Design review of the part built by this model. Coordinates are the model's own, in mm. A direction names the side the tool comes from. Give positions to 0.01 mm unless a question says otherwise; leave off trailing zeros. Order: outer loops, then holes, each group sorted by start corner. A loop starts at its lowest first (then second) coordinate and runs counter-clockwise, first axis right, second up. Notation, with made-up numbers: (34.5, 29.5) -> (67.5, 29.5) arc R21 ccw to (67.5, 40.5) -> close; hole circle Ø10 at (-9, 83.5). An arc over 180 degrees is marked (long way). One line per item, written item: value.
Autodesk Fusion 360 part; units mm, degrees
sketch "スケッチ1" plane through (0, 0, 0) normal (0, 0, 1) x (1, 0, 0)
  line L0 (0, 45) -> (0, 0)
  line L1 (4, 10.5) -> (4, 45)
  line L2 (45, 4) -> (10.5, 4)
  line L3 (0, 0) -> (45, 0)
  arc A0 (4, 10.5) -> (10.5, 4) centre (10.5, 10.5) ccw
  line L4 (45, 0) -> (45, 4)
  line L5 (4, 45) -> (0, 45)
extrude "押し出し1" add sketch "スケッチ1" along normal blind 100
Item 1: Add section B-B on x = 16.5. Give the boundary of the cut face in (y, z).
Returned:
outline: (0, 0) -> (4, 0) -> (4, 100) -> (0, 100) -> close
Item 2: To check wall thickness, follow line 1 along X through (y, z) = (26, 80); line 2 along X through (y, z) = (9, 60). State the ranges of each line that lie inside material, in increasing order. Write a range as from..to.
Returned:
line 1: 0..4
line 2: 0..4.18
Item 3: Clearance check with flat-ended pins moving along their axes: P1, Ø4, axis at x = 26, z = 62.5, coming from the +Y side; P2, Ø10.5, axis at y = 36, z = 53, coming from the +X side; P3, Ø6, axis at y = 33.5, z = 38, coming from the -X side; P4, Ø4, axis at y = 10.5, z = 58.5, coming from the +X side. State where each tip first meets the part, or that it passes through.
Returned:
P1: y = 4
P2: x = 4
P3: x = 0
P4: x = 4.32
Item 4: Machinability: for faces 1 (the flat face through (22, 0, 49)), 2 (the flat face through (28, 4, 49)), which of the approach directions +Z, -Z, +X, -X, +Y, -Y give a long, thin tool a straight path to every point of the face, cutting with its end or side? Answer none if there is none.
Returned:
face 1: +Z, -Z, +X, -X, -Y
face 2: +Z, -Z, +X, +Y
Item 5: Add section C-C on y = 5.5. Give the boundary of the cut face in (x, z).
Returned:
outline: (0, 0) -> (6.35, 0) -> (6.35, 100) -> (0, 100) -> close
Item 6: Add section A-A on z = 77.5. Give the boundary of the cut face in (x, y), plus the area to 3 significant figures.
Returned:
outline: (0, 0) -> (45, 0) -> (45, 4) -> (10.5, 4) arc R6.5 cw to (4, 10.5) -> (4, 45) -> (0, 45) -> close
area: 353 mm²
